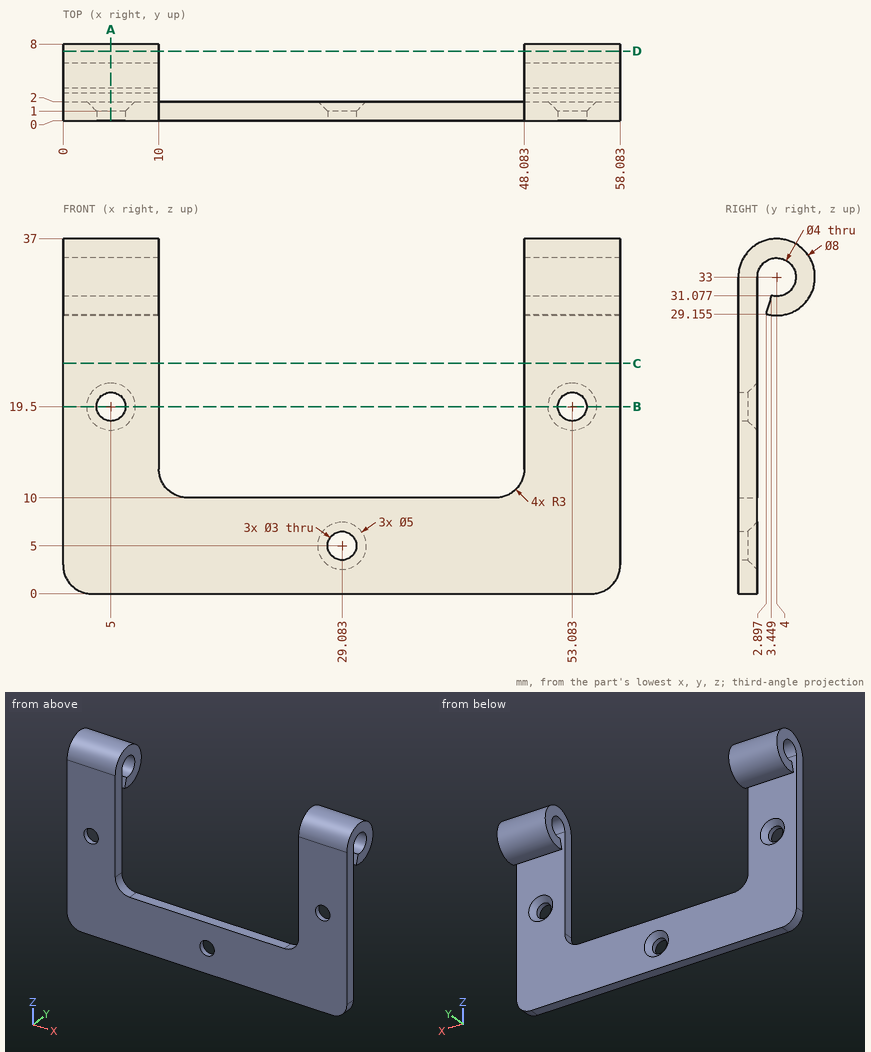
Verification items for this drawing (mm, ordinates from the low corner). Coordinates: 2 decimals unless noted, no trailing zeros. Order: outer loops, then holes, each group sorted by start corner. A loop starts at its lowest first (then second) coordinate and runs counter-clockwise, first axis right, second up. Notation, with made-up numbers: (75.25, 60) - (123.25, 60) arc R18 ccw to (123.25, 66) - close; hole circle Ø2 at (59, -23.5). An arc over 180 degrees is marked (long way). Answer as a JSON object with one key per item and string values. Group by question number.
Item 1: Sectioned sample at A-A, the plane x = 5. Record the cut outline in (y, z) (1 decimal).
Item 2: Scan lines: probe 1 along X at (y, z) = (0.35, 19.5); probe 2 along X at (y, z) = (0.55, 5); probe 3 along Y at (x, z) = (4, 33). Record each from-to range of solid material in increasing order.
Item 3: Sectioned sample at B-B, the plane z = 19.5. Record the cut outline in (x, y).
Item 4: Sectioned sample at D-D, the plane y = 7.25. Record the cut outline in (x, z).
Item 5: Sectioned sample at C-C, the plane z = 24. Record the cut outline in (x, y).
Item 6: Depth check by flat-ended pin: pin 1 Ø1 at (x, y) = (25, 0.5) entering from +Z; pin 2 Ø5 at (x, z) = (39.5, 11) entering from +Y; pin 3 Ø4 at (x, z) = (53.08, 19.5) entering from +Y (1 decimal). Enter the tip coordinate at first touch or a pass-through.
Resolved:
{
 "1": {"outline": "(0, 0) - (2, 0) - (2, 17) - (1, 18) - (0, 18) - close; (0, 21) - (1, 21) - (2, 22) - (2, 33) arc R2 cw (long way) to (3.4, 31.1) - (2.9, 29.2) arc R4 ccw (long way) to (0, 33) - close"},
 "2": {"probe 1": "0 to 3.5, 6.5 to 10, 48.08 to 51.58, 54.58 to 58.08", "probe 2": "0 to 27.58, 30.58 to 58.08", "probe 3": "0 to 2, 6 to 8"},
 "3": {"outline": "(0, 0) - (3.5, 0) - (3.5, 1) - (2.5, 2) - (0, 2) - close; (6.5, 0) - (10, 0) - (10, 2) - (7.5, 2) - (6.5, 1) - close; (48.08, 0) - (51.58, 0) - (51.58, 1) - (50.58, 2) - (48.08, 2) - close; (54.58, 0) - (58.08, 0) - (58.08, 2) - (55.58, 2) - (54.58, 1) - close"},
 "4": {"outline": "(0, 30.67) - (10, 30.67) - (10, 35.33) - (0, 35.33) - close; (48.08, 30.67) - (58.08, 30.67) - (58.08, 35.33) - (48.08, 35.33) - close"},
 "5": {"outline": "(0, 0) - (10, 0) - (10, 2) - (0, 2) - close; (48.08, 0) - (58.08, 0) - (58.08, 2) - (48.08, 2) - close"},
 "6": {"pin 1": "z = 10", "pin 2": "y = 2", "pin 3": "y = 1.5"}
}
